Can you work these out from the model? Positions are in its coordinate system, mm. Coordinates: 2 decimals unless noted, no trailing zeros. Write each loop counter-clockwise with the first axis right and the second up, starting at its lowest first coordinate (ties: lowest second). Pieces come first, ordered by that corner, then holes. Notation, with made-up numbers: (53.5, -18.5) -> (62.5, -18.5) arc R21 ccw to (62.5, 20.5) -> close; hole circle Ø10 at (-30, -19.75). An arc over 180 degrees is marked (long way). Answer as CSV lines item,"result". Start each with the question number.
```python
from build123d import *

# Parameters (mm, degrees)
BOSS_EXTRUDE1_DEPTH = 8
FILLET1_R           = 8
FILLET2_R           = 5
FILLET3_R           = 5
SKETCH2_R           = 2.5
CUT_EXTRUDE1_DEPTH  = 96.327068709


with BuildPart() as part:
    # Sketch1 → Boss-Extrude1 (new, symmetric)
    with BuildSketch(Plane.XY):
        with BuildLine():
            Line((0, 0), (0, 45))
            ThreePointArc((0, 45), (41.839723947, 41.475158976), (82.5, 31))
            Line((82.5, 31), (82.5, 13))
            Line((82.5, 13), (43.165682973, 8.697844187))
            add(Edge.make_bspline(
                [(25.5, 0), (25.5, 6.5), (43.165682973, 8.697844187)],
                knots=[0, 0, 0, 1, 1, 1], degree=2))
            Line((25.5, 0), (0, 0))
        make_face()
    boss_extrude1 = extrude(amount=BOSS_EXTRUDE1_DEPTH, both=True)

    # Mirror1: Boss-Extrude1 across plane
    add(boss_extrude1.mirror(Plane(origin=(0, 0, 0), x_dir=(0, 0, 1), z_dir=(1, 0, 0))))

    # Fillet1
    fillet1_edges = [part.edges().sort_by_distance(p)[0] for p in [
        (82.5, 31, 0),
        (-82.5, 31, 0),
    ]]
    fillet(fillet1_edges, radius=FILLET1_R)

    # Fillet2
    fillet2_edges = [part.edges().sort_by_distance(p)[0] for p in [
        (82.5, 13, 0),
        (-82.5, 13, 0),
    ]]
    fillet(fillet2_edges, radius=FILLET2_R)

    # Fillet3
    fillet3_edges = [part.edges().sort_by_distance(p)[0] for p in [
        (25.5, 0, 4),
        (-25.5, 0, -4),
    ]]
    fillet(fillet3_edges, radius=FILLET3_R)

    # Sketch2 → Cut-Extrude1 (cut, through all)
    with BuildSketch(Plane.XY.offset(8)):
        with Locations((49.5, 18)):
            Circle(SKETCH2_R)
    cut_extrude1 = extrude(amount=-CUT_EXTRUDE1_DEPTH, mode=Mode.SUBTRACT)

    # Mirror4: Cut-Extrude1 across plane
    add(cut_extrude1.mirror(Plane(origin=(0, 0, 0), x_dir=(0, 0, 1), z_dir=(1, 0, 0))), mode=Mode.SUBTRACT)


solid = part.part
```
Q1. Imagine slicing it at A-A (x = -49.5). Write out the boundary of the cut face in (y, z).
Q2. For pin 1 (6.5 mm diameter, centred on x = -49.5, y = 18, fed in from -Z); pin 2 (5 mm diameter, centred on x = 49, z = -6, fed in from +Y); pin 3 (4 mm diameter, centred on x = -52, z = 5.5, fed in from -Y), each with a flat end and sliding along its axis, tell me the tip position at first contact or that it passes through.
Q3. If we mould it in two halves opening along X, with no side actions, what happens to faces 1 (the face through (-81.257, 14.183, -0.112)), 2 (the face through (81.257, 14.183, -0.112)), 3 (the face through (-51, 20, 0))? For each: released by +X, released by -X, zero draft, split by the parting line, or undercut.
Q4. I need wall thicknesses on L1, parallel to X at y = 19.5, z = 5; L2, parallel to Y at x = -49.5, z = -3.25; L3, parallel to Y at x = 75, z = -2.25. Which ranges of each line are inside material? Lowest first, please.
Q5. Imagine slicing it at C-C (y = 36.5). Write out the boundary of the cut face in (x, z).
Q6. Imagine slicing it at B-B (z = -2.75). State how many separate pieces and enclosed holes the cut face has, then the cut area to 3 significant figures.
Entries:
1,outline,"(9.39, -8) -> (15.5, -8) -> (15.5, 8) -> (9.39, 8) -> close; (20.5, -8) -> (40.05, -8) -> (40.05, 8) -> (20.5, 8) -> close"
2,pin 1,"z = -8"
2,pin 2,"y = 40.64"
2,pin 3,"y = 9.45"
3,face 1,"released by -X"
3,face 2,"released by +X"
3,face 3,"undercut"
4,L1,"-82.5 to -51.5, -47.5 to 47.5, 51.5 to 82.5"
4,L2,"9.39 to 15.5, 20.5 to 40.05"
4,L3,"12.18 to 33.49"
5,outline,"(-64.65, -8) -> (64.65, -8) -> (64.65, 8) -> (-64.65, 8) -> close"
6,separate pieces,"1"
6,enclosed holes,"2"
6,area,"5,520 mm2"
